from build123d import *

# Parameters (mm, degrees)
SKETCH1_W            = 30
SKETCH1_H            = 30
BOSS_EXTRUDE1_DEPTH  = 2
SKETCH2_W            = 7
SKETCH2_H            = 12
CUT_EXTRUDE1_DEPTH   = 22.307275753
M4_CLEARANCE_HOLE1_D = 4.5
BOSS_EXTRUDE2_DEPTH  = 2
M5_CLEARANCE_HOLE1_D = 5.5
FILLET1_R            = 5
FILLET2_R            = 0.5


with BuildPart() as part:
    # Sketch1 → Boss-Extrude1 (new body)
    with BuildSketch(Plane(origin=(0, 0, 0), x_dir=(0, 0, -1), z_dir=(1, 0, 0))):
        Rectangle(SKETCH1_W, SKETCH1_H)
    extrude(amount=BOSS_EXTRUDE1_DEPTH)

    # Sketch2 → Cut-Extrude1 (cut, through all)
    with BuildSketch(Plane(origin=(2, 0, 0), x_dir=(0, 0, -1), z_dir=(1, 0, 0))):
        with Locations((-7, 0)):
            Rectangle(SKETCH2_W, SKETCH2_H)
        with Locations((7, 0)):
            Rectangle(SKETCH2_W, SKETCH2_H)
    extrude(amount=-CUT_EXTRUDE1_DEPTH, mode=Mode.SUBTRACT)

    # M4 Clearance Hole1 (through all)
    with Locations(Plane(origin=(2, 0, 0), x_dir=(0, 0, -1), z_dir=(1, 0, 0))):
        with Locations((-8, 8.5), (-8, -7.5), (8, 8.5), (8, -7.5)):
            Hole(M4_CLEARANCE_HOLE1_D / 2)

    # Sketch6 → Boss-Extrude2 (add)
    with BuildSketch(Plane(origin=(2, 0, 0), x_dir=(0, 0, -1), z_dir=(1, 0, 0))):
        with BuildLine():
            Line((-15, 14.258342613), (-15, 15))
            Line((-15, 15), (-9.145898034, 15))
            ThreePointArc((-9.145898034, 15), (-13.065585062, 22.464315573), (-15, 14.258342613))
        make_face()
        with BuildLine():
            Line((15, 14.258342613), (15, 15))
            Line((15, 15), (9.145898034, 15))
            ThreePointArc((9.145898034, 15), (13.065585062, 22.464315573), (15, 14.258342613))
        make_face()
        with BuildLine():
            Line((-4.031128874, -15), (4.031128874, -15))
            ThreePointArc((4.031128874, -15), (0, -21.5), (-4.031128874, -15))
        make_face()
    extrude(amount=-BOSS_EXTRUDE2_DEPTH)

    # M5 Clearance Hole1 (through all)
    with Locations(Plane(origin=(2, 0, 0), x_dir=(0, 0, -1), z_dir=(1, 0, 0))):
        with Locations((-12.5, 18), (12.5, 18), (0, -17)):
            Hole(M5_CLEARANCE_HOLE1_D / 2)

    # Fillet1
    fillet1_edges = [part.edges().sort_by_distance(p)[0] for p in [
        (1, -15, -15),
        (1, -15, 15),
        (1, 14.258342613, 15),
        (1, 15, 9.145898034),
        (1, 14.258342613, -15),
        (1, 15, -9.145898034),
        (1, -15, 4.031128874),
        (1, -15, -4.031128874),
    ]]
    fillet(fillet1_edges, radius=FILLET1_R)

    # Fillet2
    # the kernel refuses this fillet: 0.5 mm, written as the material it takes off along each edge
    with BuildSketch(Plane(origin=(4.211716771, -6, -6.322949017), x_dir=(0, 0, 1), z_dir=(-1, 0, 0))) as fillet2_piece_1:
        with BuildLine():
            CenterArc((0.884686708, -0.5), FILLET2_R, 90, 111.323686263)
            Line((0.418916219, -0.681818182), (0.409600809, -0.685454545))
            ThreePointArc((0.409600809, -0.685454545), (0.23149304, -0.327370599), (-0.00745356, -0.006666667))
            Line((-0.00745356, -0.006666667), (0, 0.01))
            Line((0, 0.01), (0.884686708, 0.01))
            Line((0.884686708, 0.01), (0.884686708, 0))
        make_face()
    extrude(amount=6.423433542, mode=Mode.SUBTRACT)
    with BuildSketch(Plane(origin=(4.057372542, -6, -9.677050983), x_dir=(0, -0.851655260409685, -0.5241023921110375), z_dir=(-1, 0, 0))) as fillet2_piece_2:
        with BuildLine():
            CenterArc((0.885636575, -0.492093973), FILLET2_R, 100.202478529, 104.477512186)
            Line((0.431309548, -0.700868859), (0.422223008, -0.705044357))
            ThreePointArc((0.422223008, -0.705044357), (0.207138222, -0.355675454), (-0.008516553, -0.005241024))
            Line((-0.008516553, -0.005241024), (0.001771273, 0.009841879))
            ThreePointArc((0.001771273, 0.009841879), (0.398536459, -0.02557712), (0.795301644, 0.009841879))
            Line((0.795301644, 0.009841879), (0.797072917, 0))
        make_face()
    extrude(amount=6.114745084, mode=Mode.SUBTRACT)
    with BuildSketch(Plane(origin=(4.057372542, -6, 9.677050983), x_dir=(0, 0, 1), z_dir=(-1, 0, 0))) as fillet2_piece_3:
        with BuildLine():
            CenterArc((0.883258668, -0.496349419), FILLET2_R, 96.927845653, 104.477512186)
            Line((0.417747823, -0.678831343), (0.408437606, -0.682480981))
            ThreePointArc((0.408437606, -0.682480981), (0.2306568, -0.326010642), (-0.00745356, -0.006666667))
            Line((-0.00745356, -0.006666667), (0, 0.01))
            ThreePointArc((0, 0.01), (0.411474508, 0.01), (0.821742824, 0.009926988))
            Line((0.821742824, 0.009926988), (0.822949017, 0))
        make_face()
    extrude(amount=6.114745084, mode=Mode.SUBTRACT)
    with BuildSketch(Plane(origin=(4.211716771, -6, 6.322949017), x_dir=(0, -0.8520285817760733, -0.5234952682084655), z_dir=(-1, 0, 0))) as fillet2_piece_4:
        with BuildLine():
            CenterArc((0.889143597, -0.492030727), FILLET2_R, 100.243314316, 111.323686264)
            Line((0.463129306, -0.753778361), (0.45460902, -0.759013314))
            Line((0.45460902, -0.759013314), (-0.008520286, -0.005234953))
            Line((-0.008520286, -0.005234953), (0.001778287, 0.009840615))
            ThreePointArc((0.001778287, 0.009840615), (0.400114618, -0.025861727), (0.79845095, 0.009840615))
            Line((0.79845095, 0.009840615), (0.800229237, 0))
        make_face()
    extrude(amount=6.423433542, mode=Mode.SUBTRACT)


solid = part.part
Read the model definition and answer for the solid it produces. Units are mm, in the model's axes. A direction names the side the tool comes from. Round coordinates to 2 decimals unless told otherwise and drop trailing zeros. Write each loop counter-clockwise with the first axis right and the second up, starting at its lowest first coordinate (ties: lowest second). Pieces come first, ordered by that corner, then holes. Notation, with made-up numbers: (62.5, 58) - (118.5, 58) arc R28 cw to (118.5, 92) - close; hole circle Ø11 at (-9, 75). An arc over 180 degrees is marked (long way). Use a Markdown table: item, result.
(1) Which of the six approach directions +Z, -Z, +X, -X, +Y, -Y give full straight-line access (tool end or side, diameter ignored) to faces 1 (the cylindrical face through (0.986, 16.08, -6.317)), 2 (the flat face through (1, -15, -9.5)), 3 (the cylindrical face through (1, -13, 14)), 4 (the flat face through (1, -6, 4))?
Reported:
| item | result |
|---|---|
| face 1 | +X, -X, +Y |
| face 2 | -Z, +X, -X, -Y |
| face 3 | +Z, +X, -X, -Y |
| face 4 | +X, -X |
(2) Each of these flat-tipped pins is pushed along its axis until it touches: pin 1 Ø0.6 at (x, y) = (1, 1.5) entering from +Z; pin 2 Ø0.8 at (x, z) = (1.5, -9.5) entering from -Y; pin 3 Ø0.6 at (x, z) = (1, 4.5) entering from +Y. Where does it stop, or does it pass through?
Reported:
| item | result |
|---|---|
| pin 1 | z = 15 |
| pin 2 | y = -15 |
| pin 3 | y = 15.26 |
(3) The part is cut by section A-A (y = 8.5). Write down the section's boundary in (x, z).
Reported:
| item | result |
|---|---|
| outline | (0, -15) - (2, -15) - (2, -10.25) - (0, -10.25) - close; (0, -5.75) - (2, -5.75) - (2, 5.75) - (0, 5.75) - close; (0, 10.25) - (2, 10.25) - (2, 15) - (0, 15) - close |
(4) The part is cut by section C-C (y = 18). Write down the section's boundary in (x, z).
Reported:
| item | result |
|---|---|
| outline | (0, -17) - (2, -17) - (2, -15.25) - (0, -15.25) - close; (0, -9.75) - (2, -9.75) - (2, -7.8) - (0, -7.8) - close; (0, 7.8) - (2, 7.8) - (2, 9.75) - (0, 9.75) - close; (0, 15.25) - (2, 15.25) - (2, 17) - (0, 17) - close |
(5) The part is cut by section D-D (z = -7). Write down the section's boundary in (x, y).
Reported:
| item | result |
|---|---|
| outline | (0, -15.42) - (2, -15.42) - (2, -9.52) - (0, -9.52) - close; (0, 6) - (2, 6) - (2, 6.48) - (0, 6.48) - close; (0, 10.52) - (2, 10.52) - (2, 16.74) - (0, 16.74) - close |
(6) The mould has two halves that part along Y. Classify faces 5 (the cylindrical face through (0.986, -15.97, -6.054)), 6 (the cylindrical face through (0.99, -9.75, 7.94)), 7 (the flat face through (0, 1, 0)): released by +Y, released by -Y, zero draft, split by the parting line, or undercut.
Reported:
| item | result |
|---|---|
| face 5 | released by -Y |
| face 6 | undercut |
| face 7 | zero draft |
(7) The part is cut by section B-B (z = 12.5). Write down the section's boundary in (x, y).
Reported:
| item | result |
|---|---|
| outline | (0, -14.33) - (2, -14.33) - (2, 15.25) - (0, 15.25) - close; (0, 20.75) - (2, 20.75) - (2, 22.5) - (0, 22.5) - close |
(8) Straight lines are drawn through the part: line 1 along Z through (x, y) = (1.7, -3.5); line 2 along Z through (x, y) = (1.25, 17.5); line 3 along Z through (x, y) = (1.05, 20). For each, find the intervals that lie inside material, in ascending order. Write a range as [from, to].
Reported:
| item | result |
|---|---|
| line 1 | [-15, -10.5], [-3.5, 3.5], [10.5, 15] |
| line 2 | [-16.97, -15.2], [-9.8, -7.54], [7.54, 9.8], [15.2, 16.97] |
| line 3 | [-16.53, -14.39], [-10.61, -8.47], [8.47, 10.61], [14.39, 16.53] |
